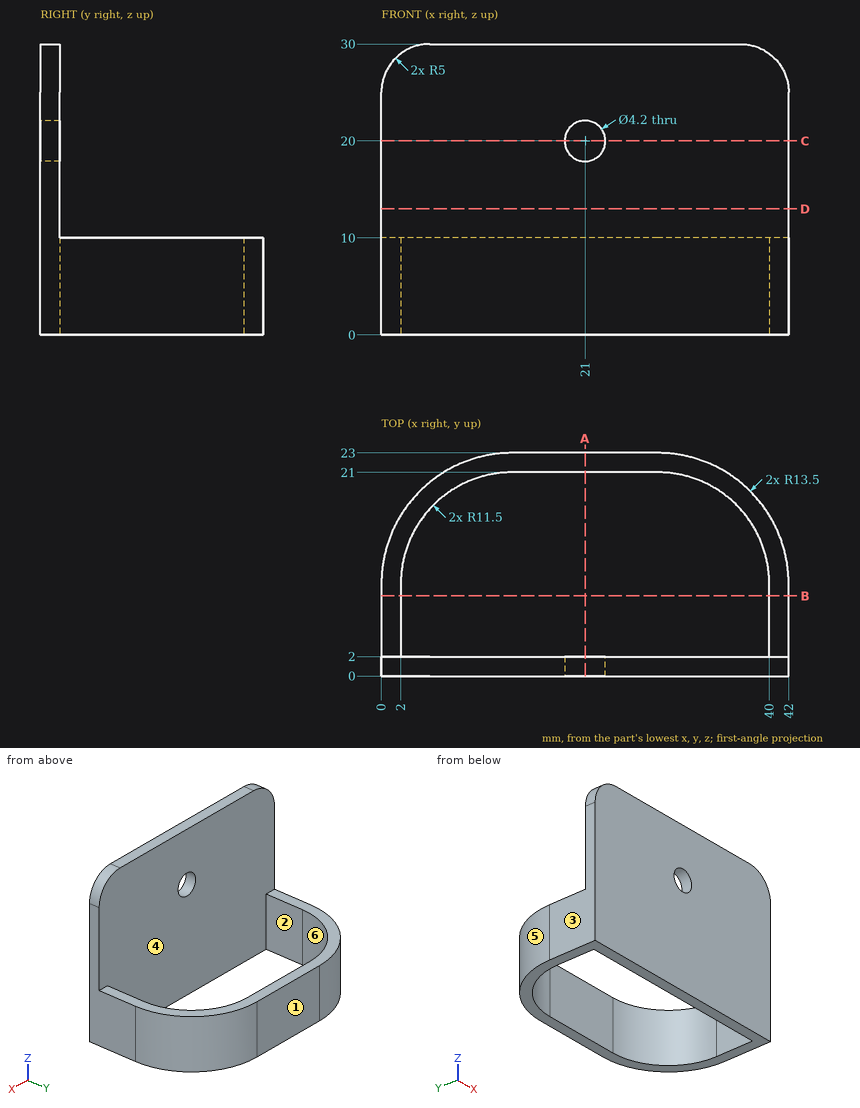
The figure shows three views and two pictorial views of one solid part (mm, origin at its lowest corner). Answer the questions. A direction names the side the tool comes from. Round coordinates to 2 decimals unless told otherwise and drop trailing zeros. Order: outer loops, then holes, each group sorted by start corner. A loop starts at its lowest first (then second) coordinate and runs counter-clockwise, first axis right, second up. Notation, with made-up numbers: (7.5, 28.5) - (27.5, 28.5) arc R34 ccw to (27.5, 62.5) - close; hole circle Ø3 at (15.25, -34). An arc over 180 degrees is marked (long way). Write item = value, one per line. Start each with the question number.
1) For a pull along Y with two mould halves and no side action, classify the marked faces 3, 4, 5 and 6 as released by +Y, released by -Y, zero draft, split by the parting line, or undercut.
2) Straight lines are drawn through the part: L1, parallel to Z at x = 21, y = 0.8; L2, parallel to Y at x = 21.5, z = 11; L3, parallel to X at y = 6.25, z = 4.5. For each, find the intervals that lie inside material, in ascending order.
3) Section B-B, the plane y = 8.25 is taken. Write down the section's boundary in (x, z).
4) Section C-C, the plane z = 20 is taken. Write down the section's boundary in (x, y), plus the area to 3 significant figures.
5) For the marked faces 1 and 2, determine the directions among +Z, -Z, +X, -X, +Y, -Y from which every point of the face is accessible in a straight line to the end or side of a thin tool.
6) Section A-A, the plane x = 21 is taken. Write down the section's boundary in (y, z).
7) Given pin 1 (6.5 mm diameter, centred on x = 14.5, y = 17, fed in from +Z); pin 2 (6 mm diameter, centred on x = 7, z = 6.5, fed in from +Y); pin 3 (1 mm diameter, centred on x = 13.5, z = 22, fed in from +Y), each flat-ended and moving along its own axis, determine where each tip first touches the part or whether it passes through.
8) Section D-D, the plane z = 13 is taken. Write down the section's boundary in (x, y), plus the area to 3 significant figures.
Results list:
q1.face_3 = zero draft
q1.face_4 = undercut
q1.face_5 = released by +Y
q1.face_6 = undercut
q2.L1 = 0 to 17.9, 22.1 to 30
q2.L2 = 0 to 2
q2.L3 = 0 to 2, 40 to 42
q3.outline = (0, 0) - (2, 0) - (2, 10) - (0, 10) - close; (40, 0) - (42, 0) - (42, 10) - (40, 10) - close
q4.outline = (0, 0) - (18.9, 0) - (18.9, 2) - (0, 2) - close; (23.1, 0) - (42, 0) - (42, 2) - (23.1, 2) - close
q4.area = 75.6 mm^2
q5.face_1 = +Z, -Z, +X, -X, +Y
q5.face_2 = +Z, -Z
q6.outline = (0, 0) - (2, 0) - (2, 17.9) - (0, 17.9) - close; (0, 22.1) - (2, 22.1) - (2, 30) - (0, 30) - close; (21, 0) - (23, 0) - (23, 10) - (21, 10) - close
q7.pin_1 = through
q7.pin_2 = 22.54
q7.pin_3 = 2
q8.outline = (0, 0) - (42, 0) - (42, 2) - (0, 2) - close
q8.area = 84.0 mm^2
